from build123d import *

# Parameters (mm, degrees)
F0_W     = 100
F0_H     = 64.25
F1_DEPTH = 5
F2_SIZE  = 5
F3_W     = 10
F3_H     = 5
F4_DEPTH = 5


# Not quite as in the source:
# - a pattern or mirror of a feature is missing from the dataset's text; its kind, count and spacing are read off the source's solid


with BuildPart() as f1:
    # F0 (on Front) → F1 (new body)
    with BuildSketch(Plane.XZ):
        Rectangle(F0_W, F0_H)
        with BuildLine():
            Line((15, -12.5), (-15, -12.5))
            ThreePointArc((-15, -12.5), (-27.5, 0), (-15, 12.5))
            Line((-15, 12.5), (15, 12.5))
            ThreePointArc((15, 12.5), (27.5, 0), (15, -12.5))
        make_face(mode=Mode.SUBTRACT)
    extrude(amount=F1_DEPTH)

    # F2
    f2_edges = [f1.edges().sort_by_distance(p)[0] for p in [
        (-50, -2.5, 32.125),
        (50, -2.5, 32.125),
        (-50, -2.5, -32.125),
        (50, -2.5, -32.125),
    ]]
    chamfer(f2_edges, length=F2_SIZE)

    # F3 (on face) → F4 (join)
    with BuildSketch(Plane(origin=(0, 0, -32.125), x_dir=(1, 0, 0), z_dir=(0, 0, -1))):
        with Locations((35, 2.5)):
            Rectangle(F3_W, F3_H)
        with Locations((15, 2.5)):
            Rectangle(F3_W, F3_H)
        with Locations((-15, 2.5)):
            Rectangle(F3_W, F3_H)
        with Locations((-35, 2.5)):
            Rectangle(F3_W, F3_H)
    f4 = extrude(amount=F4_DEPTH)

    # F4_copies: F4 across plane
    add(f4.mirror(Plane.XY))


solid = f1.part
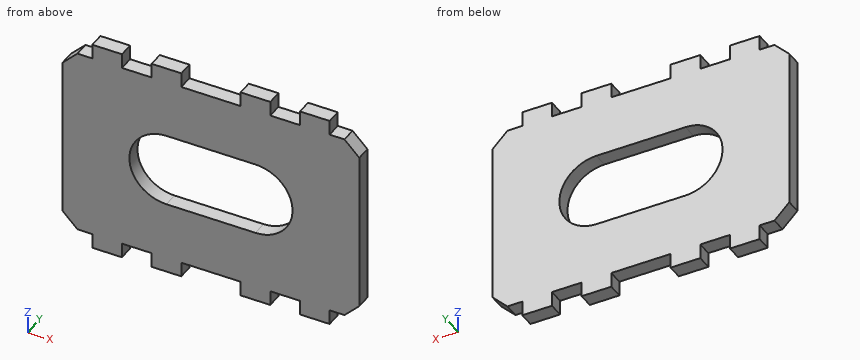
Geometry: final body of the model. Coordinates: model frame, mm. Give positions to 0.01 mm unless a question says otherwise; leave off trailing zeros. Loops run counter-clockwise (first coordinate to the right, second up) from the corner with the lowest first, then second, coordinate; pieces in that order, holes last. Notation, with made-up numbers: (54, -35) -> (87, -35) arc R24 cw to (87, -5) -> close; hole circle Ø7 at (88, 26.5). An arc over 180 degrees is marked (long way). Put each result on its own line as item: value.
1. Pin query (flat end, axial travel): P1, Ø2.5, axis at y = -2.5, z = -33.5, coming from the -X side; P2, Ø2.5, axis at y = -3, z = 33.5, coming from the +X side; P3, Ø2.5, axis at x = -4, y = -2, coming from the -Z side (3 decimals). Return the tip coordinate at first contact, or that it passes through.
Taken from the geometry:
P1: stops at x = -40
P2: stops at x = 40
P3: stops at z = -32.125
2. Cut plane A-A (x = -9). Return the cut outline in (y, z) (3 decimals).
Taken from the geometry:
outline: (-5, -32.125) -> (0, -32.125) -> (0, -12.5) -> (-5, -12.5) -> close; (-5, 12.5) -> (0, 12.5) -> (0, 32.125) -> (-5, 32.125) -> close
3. Cut plane B-B (z = 0). Return the cut outline in (x, y).
Taken from the geometry:
outline: (-50, -5) -> (-27.5, -5) -> (-27.5, 0) -> (-50, 0) -> close; (27.5, -5) -> (50, -5) -> (50, 0) -> (27.5, 0) -> close
4. Ray query, line 1 along Z through (x, y) = (8, -0.2) (3 decimals); line 2 along X through (y, z) = (-2.25, -0.5); line 3 along Z through (x, y) = (-42.5, -4.05) (3 decimals). Return the intervals inside material, ascending. Write a range as [from, to].
Taken from the geometry:
line 1: z = [-32.125, -12.5], [12.5, 32.125]
line 2: x = [-50, -27.49], [27.49, 50]
line 3: z = [-32.125, 32.125]
